from build123d import *

# Parameters (mm, degrees)
SKETCH_R        = 6
PAD_DEPTH       = 12
SKETCH001_R     = 3.1
POCKET_DEPTH    = 6
SKETCH002_R     = 1.6
POCKET001_DEPTH = 6
SKETCH003_R     = 1.85
POCKET002_DEPTH = 6.001


with BuildPart() as part:
    # Sketch → Pad (new body)
    with BuildSketch(Plane.XY):
        Circle(SKETCH_R)
    extrude(amount=PAD_DEPTH)

    # Sketch001 (on Face3 of Pad) → Pocket (cut)
    with BuildSketch(Plane.XY.offset(12)):
        Circle(SKETCH001_R)
    extrude(amount=-POCKET_DEPTH, mode=Mode.SUBTRACT)

    # Sketch002 (on Face2 of Pocket) → Pocket001 (cut)
    with BuildSketch(Plane(origin=(0, 0, 0), x_dir=(1, 0, 0), z_dir=(0, 0, -1))):
        Circle(SKETCH002_R)
    extrude(amount=-POCKET001_DEPTH, mode=Mode.SUBTRACT)

    # Sketch003 → Pocket002 (cut, through all)
    with BuildSketch(Plane.XZ):
        with Locations((0, 9)):
            Circle(SKETCH003_R)
        with Locations((0, 3)):
            Circle(SKETCH003_R)
    extrude(amount=-POCKET002_DEPTH, mode=Mode.SUBTRACT)


solid = part.part
Read the model definition and answer for the solid it produces. Units are mm, in the model's axes. A direction names the side the tool comes from. Coordinates: 2 decimals unless noted, no trailing zeros. Loops run counter-clockwise (first coordinate to the right, second up) from the corner with the lowest first, then second, coordinate; pieces in that order, holes last. Notation, with made-up numbers: (-30, 8.25) -> (14, 8.25) arc R10 ccw to (14, 18.25) -> close; hole circle Ø6 at (24, -37). An arc over 180 degrees is marked (long way). Write item = value, one per line. Start each with the question number.
1) The part is cut by section A-A, the plane x = 0. Determine the outline of the cut face in (y, z).
2) Given P1, Ø2, axis at y = 1.5, z = 4.5, coming from the -X side; P2, Ø2, axis at x = 0, z = 3, coming from the +Y side; P3, Ø1, axis at x = -1, z = 4, coming from the -Y side, each flat-ended and moving along its own axis, determine where each tip first touches the part or whether it passes through.
3) The part is cut by section D-D, the plane z = 3.5. Determine the outline of the cut face in (x, y).
4) The part is cut by section B-B, the plane y = 2.75. Determine the outline of the cut face in (x, z).
5) The part is cut by section C-C, the plane x = -2.25. Determine the outline of the cut face in (y, z).
6) The mould has two halves that part along Y. Classify faces 4 (the face through (-1.301, -5.857, 5.916)), 5 (the face through (1.71, 4.22, 8.29)), 6 (the face through (-0.672, -3.026, 9.042)): pulls with the +Y half, pulls with the -Y half, needs draft (parallel to the pull), parting line crosses it, or undercut.
7) For faces 1 (the face through (3, -3, 12)), 2 (the face through (1.765, 3.629, 3.556)), 3 (the face through (1.3, -1.3, 6)), determine the directions among +Z, -Z, +X, -X, +Y, -Y from which every point of the face is accessible in a straight line to the end or side of a thin tool.
8) Find the intervals of material crossed by L1, parallel to Z at x = 0, y = 3.35; L2, parallel to Z at x = 0, y = 2.75; L3, parallel to Y at x = 0, z = 8.75, in increasing order. Write a range as from..to.
Result:
q1.outline = (-6, 0) -> (-1.6, 0) -> (-1.6, 6) -> (-3.1, 6) -> (-3.1, 12) -> (-6, 12) -> close; (1.6, 0) -> (6, 0) -> (6, 1.15) -> (1.6, 1.15) -> close; (1.6, 4.85) -> (6, 4.85) -> (6, 7.15) -> (3.1, 7.15) -> (3.1, 6) -> (1.6, 6) -> close; (3.1, 10.85) -> (6, 10.85) -> (6, 12) -> (3.1, 12) -> close
q2.P1 = -5.98
q2.P2 = -1.25
q2.P3 = -5.98
q3.outline = (-1.78, 0) -> (-1.78, 5.73) arc R6 ccw (long way) to (1.78, 5.73) -> (1.78, 0) -> (1.6, 0) arc R1.6 cw to (-1.6, 0) -> close
q4.outline = (-5.33, 0) -> (5.33, 0) -> (5.33, 12) -> (1.43, 12) -> (1.43, 10.17) arc R1.85 cw to (1.43, 7.83) -> (1.43, 6) -> (-1.43, 6) -> (-1.43, 7.83) arc R1.85 cw to (-1.43, 10.17) -> (-1.43, 12) -> (-5.33, 12) -> close; hole circle Ø3.7 at (0, 3)
q5.outline = (-5.56, 0) -> (5.56, 0) -> (5.56, 12) -> (2.13, 12) -> (2.13, 6) -> (-2.13, 6) -> (-2.13, 12) -> (-5.56, 12) -> close
q6.face_4 = parting line crosses it
q6.face_5 = needs draft
q6.face_6 = undercut
q7.face_1 = +Z, +X, -X, +Y, -Y
q7.face_2 = +Y
q7.face_3 = +Z
q8.L1 = 0..1.15, 4.85..7.15, 10.85..12
q8.L2 = 0..1.15, 4.85..6
q8.L3 = -6..-3.1
